from build123d import *

# Parameters (mm, degrees)
F1_DEPTH = 425.5
F2_R     = 7.5
F3_DEPTH = 81
F4_R     = 7.5
F5_DEPTH = 25


# Not quite as in the source:
# - a feature names something its author has since deleted; it is built from what else it names


with BuildPart() as f1:
    # F0 (on Right) → F1 (new body, symmetric)
    with BuildSketch(Plane.YZ):
        with BuildLine():
            Line((68, 0), (0, 0))
            Line((0, 0), (0, -5))
            Line((0, -5), (65, -5))
            ThreePointArc((65, -5), (67.1213203436, -5.8786796564), (68, -8))
            Line((68, -8), (68, -50))
            Line((68, -50), (73, -50))
            Line((73, -50), (73, -5))
            ThreePointArc((73, -5), (71.5355339059, -1.4644660941), (68, 0))
        make_face()
        with BuildLine():
            Line((0, -5), (0, 0))
            Line((0, 0), (-68, 0))
            ThreePointArc((-68, 0), (-71.5355339059, -1.4644660941), (-73, -5))
            Line((-73, -5), (-73, -50))
            Line((-73, -50), (-68, -50))
            Line((-68, -50), (-68, -8))
            ThreePointArc((-68, -8), (-67.1213203436, -5.8786796564), (-65, -5))
            Line((-65, -5), (0, -5))
        make_face()
    extrude(amount=F1_DEPTH, both=True)

    # F2 (on face) → F3 (cut)
    with BuildSketch(Plane.XY):
        with BuildLine():
            Line((-349.5, 38), (-425.5, 50))
            Line((-425.5, 50), (-425.5, 0))
            Line((-425.5, 0), (-425.5, -50))
            Line((-425.5, -50), (-349.5, -38))
            ThreePointArc((-349.5, -38), (-311.5, 0), (-349.5, 38))
        make_face()
        with BuildLine():
            ThreePointArc((0, 57.5), (-7.5, 50), (0, 42.5))
            Line((0, 42.5), (0, 57.5))
        make_face()
        with BuildLine():
            Line((0, 57.5), (0, 42.5))
            ThreePointArc((0, 42.5), (5.3033008589, 44.6966991411), (7.5, 50))
            ThreePointArc((7.5, 50), (5.3033008589, 55.3033008589), (0, 57.5))
        make_face()
        with BuildLine():
            ThreePointArc((349.5, 38), (311.5, 0), (349.5, -38))
            Line((349.5, -38), (425.5, -50))
            Line((425.5, -50), (425.5, 50))
            Line((425.5, 50), (349.5, 38))
        make_face()
        with Locations((-188.9763474464, 54.7889843583)):
            Circle(F2_R)
        with Locations((263.0324065685, 54.7889843583)):
            Circle(F2_R)
        with Locations((-153.3087122573, -33.7979345426)):
            Circle(F2_R)
        with Locations((-45.0354404747, -40.2978882194)):
            Circle(F2_R)
    extrude(amount=-F3_DEPTH, mode=Mode.SUBTRACT)

    # F4 (on face) → F5 (cut)
    with BuildSketch(Plane.XZ.offset(73)):
        with Locations((-382.7857971191, -27.5)):
            Circle(F4_R)
        with Locations((382.0194303989, -27.5)):
            Circle(F4_R)
        with Locations((-230.5479198694, -27.5)):
            Circle(F4_R)
        with Locations((-74.6961683035, -27.5)):
            Circle(F4_R)
    extrude(amount=-F5_DEPTH, mode=Mode.SUBTRACT)


solid = f1.part
Verification items for the finished model (mm, model axes). A direction names the side the tool comes from. Round coordinates to 2 decimals unless told otherwise and drop trailing zeros. Loops run counter-clockwise (first coordinate to the right, second up) from the corner with the lowest first, then second, coordinate; pieces in that order, holes last. Notation, with made-up numbers: (86.5, 8.25) - (122.5, 8.25) arc R36 cw to (122.5, 45.25) - close; hole circle Ø6 at (16, 14.5). An arc over 180 degrees is marked (long way). Answer in a Markdown table with one row per item. Add a question column.
Q1. Section check C-C on y = 0. Enter the section's corners in (x, z).
Q2. Material ranges on line 1 (Y direction, x = 108.5, z = -32); line 2 (Z direction, x = 306, y = -42); line 3 (X direction, y = -22, z = -4.5), recorded low to high.
Q3. Release check for a two-part mould opening along Y. For faces 4 (the face through (6, -73, -27)), 5 (the face through (-50.563, -35.229, -2.465)), 6 (the face through (-425.5, -68.4, -17.5)) record: pulls with the +Y half, pulls with the -Y half, needs draft (parallel to the pull), parting line crosses it, or undercut.
Q4. Section check B-B on x = 182. Enter the section's corners in (y, z), plus the area to 3 significant figures.
Q5. Gauge pin test, flat ends, axial feed: pin 1 (24 mm diameter, centred on x = 0, y = 50, fed in from -Z); pin 2 (12 mm diameter, centred on x = -382.79, z = -27.5, fed in from -Y); pin 3 (12 mm diameter, centred on x = -21, y = 45, fed in from +Z); pin 4 (24 mm diameter, centred on x = -188.98, y = 54.79, fed in from -Z). Record the tip position at first contact, or that the pin passes through.
Q6. Section check A-A on z = -27.5. Enter the section's corners in (x, y).
Q7. Tool access check on faces 1 (the face through (6, 73, -28)), 2 (the face through (6, 68, -29)), 3 (the face through (-390.28, -70.54, -27.17)). Record the directions out of +Z, -Z, +X, -X, +Y, -Y that give a thin tool (end or side, any length) a straight path to the whole face; none if there is none.
Found:
| question | item | result |
|---|---|---|
| 1 | outline | (-311.5, -5) - (311.5, -5) - (311.5, 0) - (-311.5, 0) - close |
| 2 | line 1 | y = -73 to -68, 68 to 73 |
| 2 | line 2 | z = -5 to 0 |
| 2 | line 3 | x = -318.52 to 318.52 |
| 3 | face 4 | pulls with the -Y half |
| 3 | face 5 | undercut |
| 3 | face 6 | needs draft |
| 4 | outline | (-73, -50) - (-68, -50) - (-68, -8) arc R3 cw to (-65, -5) - (65, -5) arc R3 cw to (68, -8) - (68, -50) - (73, -50) - (73, -5) arc R5 ccw to (68, 0) - (-68, 0) arc R5 ccw to (-73, -5) - close |
| 4 | area | 1,170 mm² |
| 5 | pin 1 | stops at z = -5 |
| 5 | pin 2 | stops at y = 68 |
| 5 | pin 3 | stops at z = 0 |
| 5 | pin 4 | stops at z = -5.59 |
| 6 | outline | (-425.5, -73) - (-390.29, -73) - (-390.29, -68) - (-425.5, -68) - close; (-425.5, 68) - (425.5, 68) - (425.5, 73) - (-425.5, 73) - close; (-375.29, -73) - (-238.05, -73) - (-238.05, -68) - (-375.29, -68) - close; (-223.05, -73) - (-82.2, -73) - (-82.2, -68) - (-223.05, -68) - close; (-67.2, -73) - (374.52, -73) - (374.52, -68) - (-67.2, -68) - close; (389.52, -73) - (425.5, -73) - (425.5, -68) - (389.52, -68) - close |
| 7 | face 1 | +Z, -Z, +X, -X, +Y |
| 7 | face 2 | -Z, +X, -X |
| 7 | face 3 | -Y |
